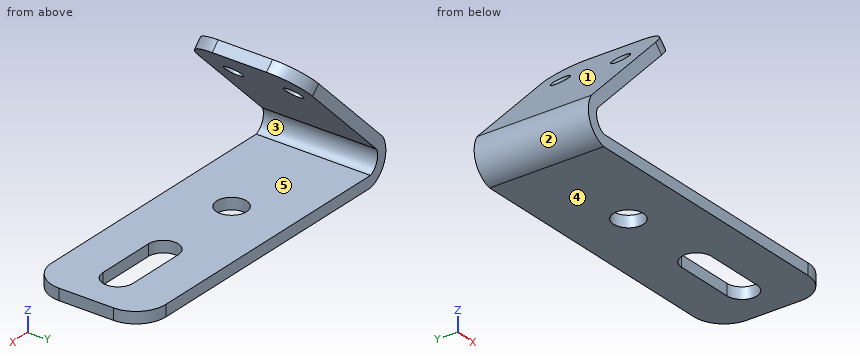
from build123d import *

# Parameters (mm, degrees)
F1_DEPTH  = 19.05
F2_R      = 5
F3_R      = 1.5
F4_DEPTH  = 10
F8_R      = 5
F9_R      = 2.5
F10_DEPTH = 25


with BuildPart() as f1:
    # F0 (on Front) → F1 (new body)
    with BuildSketch(Plane.XZ):
        with BuildLine():
            ThreePointArc((-2.7319921982, 6.5956126171), (-3.0542473294, 2.5985097523), (0, 0))
            Line((0, 0), (50, 0))
            Line((50, 0), (50, 1.9))
            Line((50, 1.9), (0, 1.9))
            ThreePointArc((0, 1.9), (-1.3800797918, 3.291972652), (-1.3884893139, 5.2521097328))
            Line((-1.3884893139, 5.2521097328), (16.2891802158, 22.9297792625))
            Line((16.2891802158, 22.9297792625), (14.9456773315, 24.2732821468))
            Line((14.9456773315, 24.2732821468), (-2.7319921982, 6.5956126171))
        make_face()
    extrude(amount=F1_DEPTH)

    # F2
    f2_edges = [f1.edges().sort_by_distance(p)[0] for p in [
        (15.617429, -19.05, 23.601531),
        (15.617429, 0, 23.601531),
    ]]
    fillet(f2_edges, radius=F2_R)

    # F3 (on face) → F4 (cut)
    with BuildSketch(Plane(origin=(-4.6638024076, 0, 4.6638024076), x_dir=(0, -1, 0), z_dir=(-0.7071067812, 0, 0.7071067812))):
        with Locations((14.55, 20.2319921982)):
            Circle(F3_R)
        with Locations((4.5, 20.2319921982)):
            Circle(F3_R)
    extrude(amount=-F4_DEPTH, mode=Mode.SUBTRACT)

    # F8
    f8_edges = [f1.edges().sort_by_distance(p)[0] for p in [
        (50, 0, 0.95),
        (50, -19.05, 0.95),
    ]]
    fillet(f8_edges, radius=F8_R)

    # F9 (on face) → F10 (cut)
    with BuildSketch(Plane.XY.offset(1.9)):
        with Locations((18, -9.525)):
            Circle(F9_R)
        with BuildLine():
            Line((33, -12.025), (43, -12.025))
            ThreePointArc((43, -12.025), (45.5, -9.525), (43, -7.025))
            Line((43, -7.025), (33, -7.025))
            ThreePointArc((33, -7.025), (30.5, -9.525), (33, -12.025))
        make_face()
    extrude(amount=-F10_DEPTH, mode=Mode.SUBTRACT)


solid = f1.part
Source: CAD feature listing. Evaluate the final solid. Frame: model axes, mm. Face numbers are marked on the shaded views. A direction names the side the tool comes from. Give positions to 0.01 mm unless a question says otherwise; leave off trailing zeros. Write each loop counter-clockwise with the first axis right and the second up, starting at its lowest first coordinate (ties: lowest second). Pieces come first, ordered by that corner, then holes. Notation, with made-up numbers: M 20,70 L 29,70 A32 ccw 29,102 Z; hole C 42,-35.75 d6. An arc over 180 degrees is marked long. Return JSON: item names as keys, results as strings. Group by question number.
1) Cut plane D-D, the plane z = 6. Output: boundary loops of the cut face in (x, y), then the cut area to 3 significant figures.
2) Draft query along Z for the marked faces 1, 2 and 3. Return one class per face: released by +Z, released by -Z, zero draft, split by the parting line, or undercut.
3) Ray query, L1, parallel to Y at x = 18, z = 0.7 (3 decimals); L2, parallel to Z at x = 22.5, y = -6; L3, parallel to Z at x = 8, y = -13.5. Return the intervals inside material, ascending.
4) Cut plane A-A, the plane x = 18. Output: boundary loops of the cut face in (y, z) (3 decimals).
5) Cut plane B-B, the plane y = -4. Output: boundary loops of the cut face in (x, z).
6) Set-up query: the marked faces 4 and 5. Return all of +Z, -Z, +X, -X, +Y, -Y with unobstructed straight access to the full face (end or side cutting, diameter ignored); none if empty.
7) First-contact query: pin 1 Ø8 at (y, z) = (-4, 15) entering from -X; pin 2 Ø4.5 at (x, y) = (18, -9.525) entering from +Z; pin 3 Ø4 at (x, y) = (3, -9) entering from +Z. Flat tips, straight axial feed; report the tip coordinate or a pass-through.
8) Cut plane C-C, the plane x = 28. Output: boundary loops of the cut face in (y, z), then the cut area to 3 significant figures.
Data:
{
 "1": {"outline": "M -3.04,-19.05 L -0.64,-19.05 L -0.64,0 L -3.04,0 Z", "area": "45.7 mm²"},
 "2": {"face 1": "released by +Z", "face 2": "split by the parting line", "face 3": "undercut"},
 "3": {"L1": "y = -19.05 to -12.025, -7.025 to 0", "L2": "z = 0 to 1.9", "L3": "z = 0 to 1.9, 14.64 to 17.33"},
 "4": {"outline": "M -19.05,0 L -12.025,0 L -12.025,1.9 L -19.05,1.9 Z; M -7.025,0 L 0,0 L 0,1.9 L -7.025,1.9 Z"},
 "5": {"outline": "M -2.73,6.6 A4.4 ccw 0,0 L 49.9,0 L 49.9,1.9 L 0,1.9 A2.59 cw -1.39,5.25 L 9.99,16.63 L 8.64,17.97 Z; M 10.64,19.97 L 11.99,18.63 L 16.22,22.86 L 14.87,24.2 Z"},
 "6": {"face 4": "-Z, +X, -X, +Y, -Y", "face 5": "+X, +Y, -Y"},
 "7": {"pin 1": "stops at x = 1.67", "pin 2": "stops at z = 23.47", "pin 3": "stops at z = 14.33"},
 "8": {"outline": "M -19.05,0 L 0,0 L 0,1.9 L -19.05,1.9 Z", "area": "36.2 mm²"}
}
